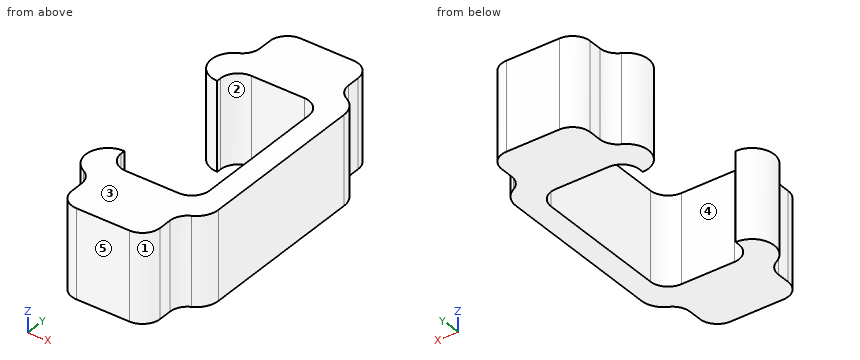
from build123d import *

# Parameters (mm, degrees)
F1_DEPTH = 25.4
F2_R     = 5.08
F3_DEPTH = 12.7
F4_DEPTH = 12.7
F5_R     = 5.08


with BuildPart() as f1:
    # F0 (on Top) → F1 (new body)
    with BuildSketch(Plane.XY):
        with BuildLine():
            Line((-24.6420629978, 11.6016305983), (-30.9920629978, 11.6016305983))
            ThreePointArc((-30.9920629978, 11.6016305983), (-29.1321910584, 7.1115025378), (-24.6420629978, 5.2516305983))
            ThreePointArc((-24.6420629978, 5.2516305983), (-20.1519349373, 7.1115025378), (-18.2920629978, 11.6016305983))
            Line((-18.2920629978, 11.6016305983), (-18.2920629978, 60.1065419614))
            ThreePointArc((-18.2920629978, 60.1065419614), (-20.1519349373, 64.596670022), (-24.6420629978, 66.4565419614))
            Line((-24.6420629978, 66.4565419614), (-50.0420629978, 66.4565419614))
            ThreePointArc((-50.0420629978, 66.4565419614), (-56.3920629978, 60.1065419614), (-50.0420629978, 53.7565419614))
            Line((-50.0420629978, 53.7565419614), (-50.0420629978, 60.1065419614))
            Line((-50.0420629978, 60.1065419614), (-24.6420629978, 60.1065419614))
            Line((-24.6420629978, 60.1065419614), (-24.6420629978, 11.6016305983))
        make_face()
        with BuildLine():
            Line((-30.9920629978, 11.6016305983), (-50.0420629978, 11.6016305983))
            Line((-50.0420629978, 11.6016305983), (-50.0420629978, 17.9516305983))
            ThreePointArc((-50.0420629978, 17.9516305983), (-56.3920629978, 11.6016305983), (-50.0420629978, 5.2516305983))
            Line((-50.0420629978, 5.2516305983), (-24.6420629978, 5.2516305983))
            ThreePointArc((-24.6420629978, 5.2516305983), (-29.1321910584, 7.1115025378), (-30.9920629978, 11.6016305983))
        make_face()
    extrude(amount=F1_DEPTH)

    # F2
    f2_edges = [f1.edges().sort_by_distance(p)[0] for p in [
        (-24.642063, 11.601631, 12.7),
        (-24.642063, 60.106542, 12.7),
        (-50.042063, 60.106542, 12.7),
        (-50.042063, 11.601631, 12.7),
    ]]
    fillet(f2_edges, radius=F2_R)

    # F3 (add): a face of the model
    f3_faces = [f1.faces().sort_by_distance(p)[0] for p in [
        (-37.3420629978, 66.4565419614, 12.7),
    ]]
    extrude(f3_faces, amount=F3_DEPTH)

    # F4 (add): a face of the model
    f4_faces = [f1.faces().sort_by_distance(p)[0] for p in [
        (-37.3420629978, 5.2516305983, 12.7),
    ]]
    extrude(f4_faces, amount=F4_DEPTH)

    # F5
    f5_edges = [f1.edges().sort_by_distance(p)[0] for p in [
        (-50.042063, 79.156542, 12.7),
        (-50.042063, -7.448369, 12.7),
        (-50.042063, 5.251631, 12.7),
        (-50.042063, 66.456542, 12.7),
        (-24.642063, 66.456542, 12.7),
        (-24.642063, 79.156542, 12.7),
        (-24.642063, -7.448369, 12.7),
        (-24.642063, 5.251631, 12.7),
    ]]
    fillet(f5_edges, radius=F5_R)


solid = f1.part
Input: part model. Units: mm. Frame: model coordinates. Face numbers are marked on the shaded views. A direction names the side the tool comes from. Coordinates: 2 decimals unless noted, no trailing zeros. Write each loop counter-clockwise with the first axis right and the second up, starting at its lowest first coordinate (ties: lowest second). Pieces come first, ordered by that corner, then holes. Notation, with made-up numbers: M 88,21.25 L 118,21.25 A30 cw 118,52.25 Z; hole C 59.5,-10 d10. An arc over 180 degrees is marked long. Answer as a JSON object with one key per item and string values. Group by question number.
(1) Section B-B on y = 56.5. Output: boundary loops of the cut face in (x, z).
(2) Mould query, pull axis Y, two halves, no side actions, for the marked faces 3, 4 and 5. Classes: pulls with the +Y half, pulls with the -Y half, needs draft (parallel to the pull), parting line crosses it, or undercut.
(3) Section A-A on x = -32. Output: boundary loops of the cut face in (y, z), plus the area to 3 significant figures.
(4) Set-up query: the marked faces 1 and 2. Return all of +Z, -Z, +X, -X, +Y, -Y with unobstructed straight access to the full face (end or side cutting, diameter ignored); none if empty.
(5) Contact query for flat-ended pins moving along their axis: P1, Ø1.1, axis at y = -0.5, z = 15.5, coming from the -X side; P2, Ø8, axis at y = 3, z = 4.5, coming from the -X side; P3, Ø1.9, axis at y = 72.5, z = 8.5, coming from the +X side. Output: stop coordinate, or through.
(6) Section C-C on z = 17.5. Output: boundary loops of the cut face in (x, y), plus the area to 3 significant figures.
(7) Ray query, line 1 along Y through (x, z) = (-35.5, 13.5); line 2 along X through (y, z) = (18.5, 5.5); line 3 along Y through (x, z) = (-55, 8.5). Return the intervals inside material, ascending. Write a range as [from, to].
(8) Section D-D on y = 68. Output: boundary loops of the cut face in (x, z), plus the area to 3 significant figures.
Result set:
{
 "1": {"outline": "M -55.27,0 L -49.82,0 L -49.82,25.4 L -55.27,25.4 Z; M -24.86,0 L -18.29,0 L -18.29,25.4 L -24.86,25.4 Z"},
 "2": {"face 3": "needs draft", "face 4": "undercut", "face 5": "pulls with the -Y half"},
 "3": {"outline": "M -7.45,0 L 11.6,0 L 11.6,25.4 L -7.45,25.4 Z; M 60.11,0 L 79.16,0 L 79.16,25.4 L 60.11,25.4 Z", "area": "968 mm2"},
 "4": {"face 1": "+Z, -Z, +X, -Y", "face 2": "+Z, -Z"},
 "5": {"P1": "stops at x = -50.04", "P2": "stops at x = -54.42", "P3": "stops at x = -24.64"},
 "6": {"outline": "M -52.86,5.91 A5.08 cw -50.04,1.36 L -50.04,-2.37 A5.08 ccw -44.96,-7.45 L -29.72,-7.45 A5.08 ccw -24.64,-2.37 L -24.64,1.36 A5.08 cw -21.82,5.91 A6.35 ccw -18.29,11.6 L -18.29,60.11 A6.35 ccw -21.82,65.79 A5.08 cw -24.64,70.35 L -24.64,74.08 A5.08 ccw -29.72,79.16 L -44.96,79.16 A5.08 ccw -50.04,74.08 L -50.04,70.35 A5.08 cw -52.86,65.79 A6.35 ccw -50.04,53.76 L -50.04,55.03 A5.08 cw -44.96,60.11 L -29.72,60.11 A5.08 cw -24.64,55.03 L -24.64,16.68 A5.08 cw -29.72,11.6 L -44.96,11.6 A5.08 cw -50.04,16.68 L -50.04,17.95 A6.35 ccw Z", "area": "1,480 mm2"},
 "7": {"line 1": "y = [-7.45, 11.6], [60.11, 79.16]", "line 2": "x = [-24.64, -18.29]", "line 3": "y = [7.63, 15.57], [56.14, 64.07]"},
 "8": {"outline": "M -50.62,0 L -24.07,0 L -24.07,25.4 L -50.62,25.4 Z", "area": "674 mm2"}
}
